Geometry: final body of the model. Coordinates: model frame, mm. A direction names the side the tool comes from. Give positions to 0.01 mm unless a question says otherwise; leave off trailing zeros. Write each loop counter-clockwise with the first axis right and the second up, starting at its lowest first coordinate (ties: lowest second). Pieces come first, ordered by that corner, then holes. Notation, with made-up numbers: (81, 35) -> (116, 35) arc R20 cw to (116, 43) -> close; hole circle Ø3 at (66, -37). An arc over 180 degrees is marked (long way). Answer in a Markdown table with one row per item. Add a question column.
Item 1: Section query A-A on z = 2.5. Output: boundary loops of the cut face in (x, y) (1 decimal).
Item 2: Draft query along Y for faces 4 (the flat face through (27.463, -1.154, 5.916)), 5 (the flat face through (50, -10.6, 6)), 6 (the flat face through (25, -8, 12)). Return one class per face: +Y half, -Y half, draft (parallel to the pull), parting line (faces both ways), or undercut.
Item 3: Section query D-D on y = -9.5. Output: boundary loops of the cut face in (x, z).
Item 4: Access query for faces 1 (the flat face through (12.48, -1.41, 5.92)), 2 (the flat face through (42.728, -8, 6)), 3 (the flat face through (51.228, -13, 6)). Directions: +Z, -Z, +X, -X, +Y, -Y. A direction counts if a zero-diameter tool reaches every point of the face in a straight line with its end or side. Return the directions, or none.
Item 5: Section query B-B on y = -4. Output: boundary loops of the cut face in (x, z).
Item 6: First-contact query: P1, Ø0.8, axis at y = -11, z = 6, coming from the -X side; P2, Ø3, axis at x = 12.5, z = 7.5, coming from the +Y side; P3, Ø1.5, axis at x = 5.5, z = 7, coming from the +Y side. Flat tips, straight axial feed; report the tip coordinate or a pass-through.
Item 7: Material intervals for probe 1 along X at (y, z) = (-4.5, 5.5); probe 2 along Y at (x, z) = (44, 4) (3 decimals); probe 3 along X at (y, z) = (-11.5, 6.75), sorted ascending. Write a range as from..to.
Item 8: Section query C-C on x = 13. Output: boundary loops of the cut face in (y, z).
Autodesk Inventor part; units mm, degrees
ref_plane "YZ Plane" through (0, 0, 0) normal (1, 0, 0) x (0, 1, 0)
ref_plane "XZ Plane" through (0, 0, 0) normal (0, 1, 0) x (-1, 0, 0)
ref_plane "XY Plane" through (0, 0, 0) normal (0, 0, 1) x (1, 0, 0)
sketch "Sketch5" plane through (0, 0, 0) normal (0, 0, 1) x (1, 0, 0)
  line L0 (51.2279, -15.6) -> (51.2279, -10.6)
  line L1 (51.2279, -10.6) -> (48.7279, -10.6)
  line L2 (48.7279, -10.6) -> (48.7279, -12.625)
  line L3 (42.7279, -12.625) -> (42.7279, -2.975)
  line L4 (48.7279, -2.975) -> (48.7279, -5)
  line L5 (48.7279, -5) -> (51.2279, -5)
  line L6 (51.2279, -5) -> (51.2279, 0)
  line L7 (42.7279, -2.975) -> (48.7279, -2.975)
  line L8 (42.7279, -12.625) -> (48.7279, -12.625)
  line L9 (51.2279, -15.6) -> (43.6357, -15.6)
  line L10 (39.8786, -15.6) -> (43.6357, -15.6)
  line L11 (0, -15.6) -> (39.8786, -15.6)
  line L12 (36.9909, 0) -> (51.2279, 0)
  line L13 (0, -15.6) -> (0, -5.4692)
  line L14 (36.9909, 0) -> (31.0226, 0)
  line L15 (0, 0) -> (0, -5.4692)
  line L16 (34.0067, 0) -> (20.7329, -2.3405)
  line L17 (0, 0) -> (20.7329, -2.3405)
  point P0 (44.1094, 0)
  dimension "d41" = 6
  dimension "d50" = 2.5
  dimension "d87" = 5.6
  dimension "d88" = 9.65
  dimension "d122" = 14.237
  dimension "d123" = 2.975
  dimension "d132" = 10
extrude "Extrusion2" add sketch "Sketch5" along normal blind 12
sketch "Sketch11" plane through (0, 0, 12) normal (0, 0, 1) x (1, 0, 0)
  line L0 (42.7279, -2.975) -> (48.7279, -2.975)
  circle A0 centre (42.7279, -2.975) radius 0.5
  line L1 (42.7279, -12.625) -> (42.7279, -2.975)
  circle A1 centre (42.7279, -12.625) radius 0.5
  line L2 (48.7279, -12.625) -> (42.7279, -12.625)
  circle A2 centre (48.7279, -12.625) radius 0.5
  line L3 (48.7279, -2.975) -> (48.7279, -5)
  circle A3 centre (48.7279, -2.975) radius 0.5
  point P0 (0, 0)
  dimension "d99" = 1
  dimension "d100" = 1
  dimension "d101" = 1
  dimension "d102" = 1
extrude "Extrusion7" cut sketch "Sketch11" against normal through all
fillet "Rundung4" radius 8 1 edges at (0, -15.6, 6)
sketch "Skizze13" plane through (0, 0, 0) normal (-1, 0, 0) x (0, 0, 1)
  point P0 (0, 0)
fillet "Rundung6" radius 4 1 edges at (0, 0, 6)
equation "\"l1\" = 8"
properties part number "Maria_Greifer_Dreieck2_3D-Druck"
Findings below:
| question | item | result |
|---|---|---|
| 1 | outline | (0, -7.6) arc R8 ccw to (8, -15.6) -> (51.2, -15.6) -> (51.2, -10.6) -> (48.7, -10.6) -> (48.7, -12.1) arc R0.5 cw (long way) to (48.2, -12.6) -> (43.2, -12.6) arc R0.5 cw (long way) to (42.7, -12.1) -> (42.7, -3.5) arc R0.5 cw (long way) to (43.2, -3) -> (48.2, -3) arc R0.5 cw (long way) to (48.7, -3.5) -> (48.7, -5) -> (51.2, -5) -> (51.2, 0) -> (34, 0) -> (20.7, -2.3) -> (4.4, -0.5) arc R4 ccw to (0, -4.5) -> close |
| 2 | face 4 | +Y half |
| 2 | face 5 | undercut |
| 2 | face 6 | draft |
| 3 | outline | (0.23, 0) -> (42.73, 0) -> (42.73, 12) -> (0.23, 12) -> close |
| 4 | face 1 | +Z, -Z, +Y |
| 4 | face 2 | +Z, -Z |
| 4 | face 3 | +Z, -Z, +X, +Y, -Y |
| 5 | outline | (0.03, 0) -> (42.73, 0) -> (42.73, 12) -> (0.03, 12) -> close; (48.73, 0) -> (51.23, 0) -> (51.23, 12) -> (48.73, 12) -> close |
| 6 | P1 | stops at x = 0.58 |
| 6 | P2 | stops at y = -1.24 |
| 6 | P3 | stops at y = -0.54 |
| 7 | probe 1 | x = 0..42.73, 48.73..51.23 |
| 7 | probe 2 | y = -15.6..-12.625, -2.975..0 |
| 7 | probe 3 | x = 1.02..42.73, 48.73..51.23 |
| 8 | outline | (-15.6, 0) -> (-1.47, 0) -> (-1.47, 12) -> (-15.6, 12) -> close |
